from build123d import *

# Parameters (mm, degrees)
F1_DEPTH      = 21
F6_DEPTH      = 11.6432544745
F6_DEPTH_BACK = 13.1294997266
F7_W          = 22
F7_H          = 5
F8_DEPTH      = 21.001


with BuildPart() as f1:
    # F0 (on Right) → F1 (new body)
    with BuildSketch(Plane.YZ):
        Polygon((0, 22), (0, 0), (22, 0), (13, 22), align=None)
    extrude(amount=F1_DEPTH)

    # F5 (on line) → F6 (cut, two sides)
    with BuildSketch(Plane(origin=(0, -1.3722109533, 10.0628803245), x_dir=(1, 0, 0), z_dir=(0, 0.1351132047, -0.990830168))) as f6_sk:
        with BuildLine():
            ThreePointArc((8.75, -6.9358111763), (10.5, -8.6858111763), (12.25, -6.9358111763))
            ThreePointArc((12.25, -6.9358111763), (10.5, -5.1858111763), (8.75, -6.9358111763))
        make_face()
    extrude(amount=-F6_DEPTH, mode=Mode.SUBTRACT)
    extrude(f6_sk.sketch, amount=F6_DEPTH_BACK, mode=Mode.SUBTRACT)

    # F7 (on Right) → F8 (cut, through all)
    with BuildSketch(Plane.YZ):
        with Locations((11, 2.5)):
            Rectangle(F7_W, F7_H)
    extrude(amount=F8_DEPTH, mode=Mode.SUBTRACT)


with BuildPart() as f1_1:
    # F9: moved
    add(f1.part.moved(Location((0, 0, -5))))


solid = f1_1.part
Check sheet for the modelled part. Datum: model origin and axes. Units: mm. Round coordinates to 2 decimals unless told otherwise and drop trailing zeros. Write each loop counter-clockwise with the first axis right and the second up, starting at its lowest first coordinate (ties: lowest second). Pieces come first, ordered by that corner, then holes. Notation, with made-up numbers: (85, 64.5) -> (131, 64.5) arc R11 cw to (131, 78.5) -> close; hole circle Ø1 at (-1.5, 68). An arc over 180 degrees is marked (long way). Answer as CSV lines item,"result". Start each with the question number.
1) Material ranges on line 1 (X direction, y = 4.75, z = 8.5); line 2 (Y direction, x = 11, z = 6); line 3 (X direction, y = 4.5, z = 7.25), recorded low to high. Write a range as from..to.
2) Go/stop test with flat-tipped pins: P1, Ø5, axis at x = 14, z = 12, coming from the +Y side; P2, Ø4, axis at x = 2.5, y = 15.5, coming from the +Z side. Record where each tip stops, or that it passes through.
3) Section check C-C on y = 17.25. Enter the section's corners in (x, z).
4) Section check A-A on x = 11.75. Enter the section's corners in (y, z).
5) Section check B-B on x = 3. Enter the section's corners in (y, z), and give its area (3 significant figures).
6) Release check for a two-part mould opening along Z. For faces 1 (the flat face through (0, 8, 9)), 2 (the flat face through (10.353, 16.526, 8.381)), 3 (the cylindrical face through (12.117, 5.84, 8.468)), 4 (the flat face through (10, 10, 0)) record: pulls with the +Z half, pulls with the -Z half, needs draft (parallel to the pull), parting line crosses it, or undercut.
Found:
1,line 1,"x = 0..8.8, 12.2..21"
1,line 2,"y = 0..3.81, 7.19..17.5"
1,line 3,"x = 0..8.96, 12.04..21"
2,P1,"stops at y = 16.07"
2,P2,"stops at z = 15.78"
3,outline,"(0, 0) -> (21, 0) -> (21, 6.61) -> (0, 6.61) -> close"
4,outline,"(0, 0) -> (5.08, 0) -> (2.76, 17) -> (0, 17) -> close; (5.24, 17) -> (7.55, 0) -> (19.95, 0) -> (13, 17) -> close"
5,outline,"(0, 0) -> (19.95, 0) -> (13, 17) -> (0, 17) -> close"
5,area,"280 mm^2"
6,face 1,"needs draft"
6,face 2,"pulls with the +Z half"
6,face 3,"undercut"
6,face 4,"pulls with the -Z half"
